```python
from build123d import *

# Parameters (mm, degrees)
BOSS_EXTRUDE1_DEPTH = 1.2
BOSS_EXTRUDE2_DEPTH = 3


with BuildPart() as part:
    # Sketch1 → Boss-Extrude1 (new body)
    with BuildSketch(Plane.XY):
        Polygon((0.866929529, 10.79891165), (24.866929529, 20.098165538), (24.866929529, -20.133015932), (0.866929529, -10.833762045), align=None)
    extrude(amount=BOSS_EXTRUDE1_DEPTH)

    # Sketch2 → Boss-Extrude2 (add)
    with BuildSketch(Plane(origin=(0, 0, 0), x_dir=(-1, 0, 0), z_dir=(0, 0, -1))):
        Polygon((-24.866929529, 19.789566237), (-22.866929529, 19.323227714), (-22.866929529, -19.358078108), (-24.866929529, -20.133015932), (-32.866929529, -20.133015932), (-32.866929529, -9.592041142), (-24.866929529, -9.592041142), (-24.866929529, 11.407958858), (-32.866929529, 11.407958858), (-32.866929529, 19.789566237), align=None)
    extrude(amount=-BOSS_EXTRUDE2_DEPTH)


solid = part.part
```
Input: part model. Units: mm. Frame: model coordinates. A direction names the side the tool comes from. Give positions to 0.01 mm unless a question says otherwise; leave off trailing zeros. Order: outer loops, then holes, each group sorted by start corner. A loop starts at its lowest first (then second) coordinate and runs counter-clockwise, first axis right, second up.
1. Section D-D on z = 2.4. Return the cut outline in (x, y).
Derived:
outline: (22.87, -19.36) - (24.87, -20.13) - (32.87, -20.13) - (32.87, -9.59) - (24.87, -9.59) - (24.87, 11.41) - (32.87, 11.41) - (32.87, 19.79) - (24.87, 19.79) - (22.87, 19.32) - close
2. Reachability of faces 1 (the flat face through (22.867, 0, 2)), 2 (the flat face through (23.88, 19.56, 2.09)), 3 (the flat face through (29, 19.79, 1)), 4 (the flat face through (17, 0, 0)), 5 (the flat face through (29, -9.592, 1)) from +Z, -Z, +X, -X, +Y, -Y: full face, straight path, thin tool, end or side. Return the list, or none.
Derived:
face 1: +Z, -X, +Y, -Y
face 2: +Z, -X, +Y
face 3: +Z, -Z, +X, +Y
face 4: -Z, +X, -X, +Y, -Y
face 5: +Z, -Z, +X
3. Section C-C on y = -6.5. Return the cut outline in (x, z).
Derived:
outline: (0.87, 0) - (24.87, 0) - (24.87, 3) - (22.87, 3) - (22.87, 1.2) - (0.87, 1.2) - close
4. Pin query (flat end, axial travel): pin 1 (2 mm diameter, centred on x = 18.5, y = 4, fed in from +Z); pin 2 (3 mm diameter, centred on x = 28, y = 7.5, fed in from +Z); pin 3 (1.5 mm diameter, centred on x = 29.5, z = 1.5, fed in from +Y); pin 4 (0.9 mm diameter, centred on y = -2, z = 1.5, fed in from +X). Return the tip coordinate at first contact, or that it passes through.
Derived:
pin 1: stops at z = 1.2
pin 2: passes through
pin 3: stops at y = 19.79
pin 4: stops at x = 24.87
5. Section A-A on x = 26. Return the cut outline in (y, z).
Derived:
outline: (-20.13, 0) - (-9.59, 0) - (-9.59, 3) - (-20.13, 3) - close; (11.41, 0) - (19.79, 0) - (19.79, 3) - (11.41, 3) - close
6. Mould query, pull axis Y, two halves, no side actions, for faces 6 (the flat face through (29, -20.133, 1)), 7 (the flat face through (24.867, 1, 1)), 8 (the flat face through (0.867, 0, 1)). Classes: released by +Y, released by -Y, zero draft, split by the parting line, or undercut.
Derived:
face 6: released by -Y
face 7: undercut
face 8: zero draft
7. Section B-B on z = 0.45. Return the cut outline in (x, y), and give its area (3 significant figures).
Derived:
outline: (0.87, -10.83) - (24.87, -20.13) - (32.87, -20.13) - (32.87, -9.59) - (24.87, -9.59) - (24.87, 11.41) - (32.87, 11.41) - (32.87, 19.79) - (24.87, 19.79) - (24.87, 20.1) - (0.87, 10.8) - close
area: 894 mm2
8. Material intervals for L1, parallel to Y at x = 26.5, z = 0.9; L2, parallel to Z at x = 21, y = -13; L3, parallel to X at y = 7, z = 1.55, sorted ascending.
Derived:
L1: y = -20.13 to -9.59, 11.41 to 19.79
L2: z = 0 to 1.2
L3: x = 22.87 to 24.87
